Here's the drawing with two shaded views (mm, measured from the low corner). I have some questions. Coordinates: 2 decimals unless noted, no trailing zeros. Write each loop counter-clockwise with the first axis right and the second up, starting at its lowest first coordinate (ties: lowest second). Pieces come first, ordered by that corner, then holes.
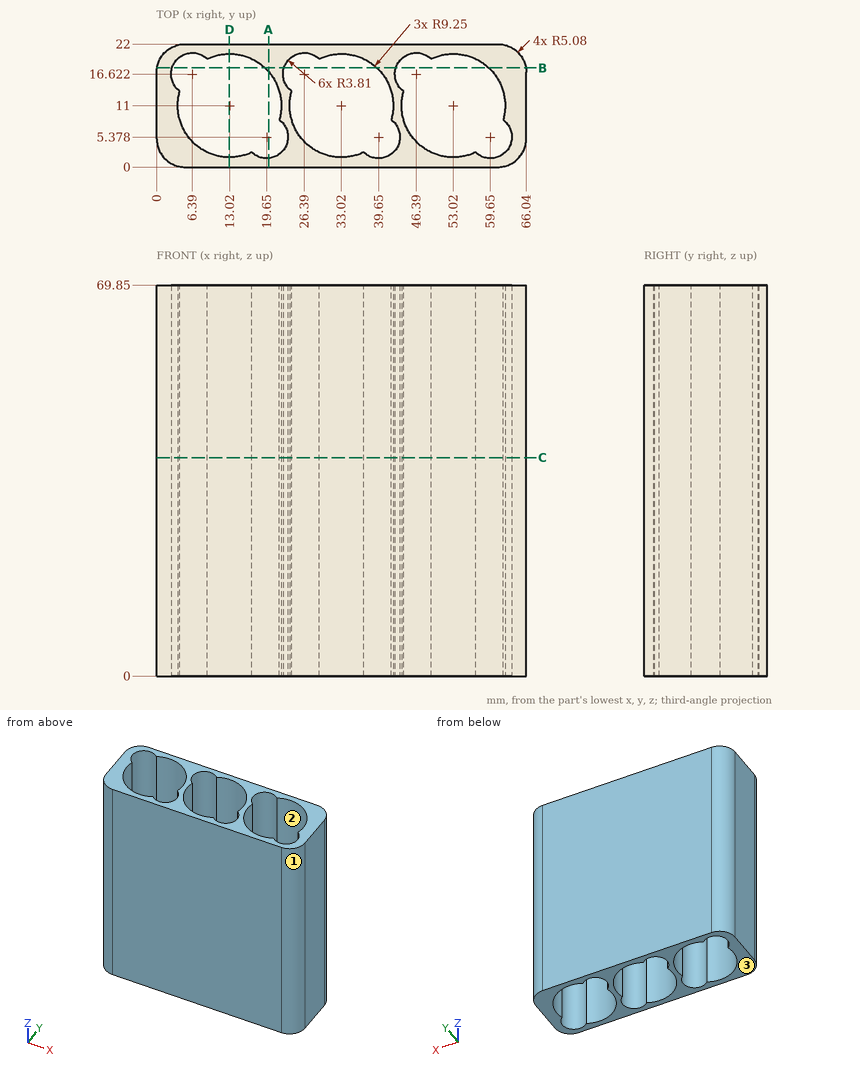
Item 1: I want a section at D-D, the plane x = 13. List the corners of the cut face in (y, z) for me.
Item 2: I want a section at A-A, the plane x = 20. List the corners of the cut face in (y, z) for me, then the cut area to 3 significant figures.
Item 3: If we mould it in two halves opening along X, with no side actions, what happens to the marked faces 1, 2 and 3? For each: released by +X, released by -X, zero draft, split by the parting line, or undercut.
Item 4: I want a section at C-C, the plane z = 39. List the corners of the cut face in (x, y) for me, then the cut area to 3 significant figures.
Item 5: I want a section at B-B, the plane y = 17.75. List the corners of the cut face in (x, z) for me, then the cut area to 3 significant figures.
Item 6: If I drill on line 1 along X through (y, z) = (10.75, 20.5); line 2 along X through (y, z) = (13.5, 38.5); line 3 along Y through (x, z) = (33, 34.5), over which ranges is the centre line in solid material (lowest first)?
Taken from the geometry:
1. outline: (0, 0) - (1.75, 0) - (1.75, 69.85) - (0, 69.85) - close; (20.25, 0) - (22, 0) - (22, 69.85) - (20.25, 69.85) - close
2. outline: (0, 0) - (1.58, 0) - (1.58, 69.85) - (0, 69.85) - close; (17.07, 0) - (22, 0) - (22, 69.85) - (17.07, 69.85) - close
2. area: 455 mm2
3. face 1: released by +X
3. face 2: undercut
3. face 3: zero draft
4. outline: (0, 5.08) arc R5.08 ccw to (5.08, 0) - (60.96, 0) arc R5.08 ccw to (66.04, 5.08) - (66.04, 16.92) arc R5.08 ccw to (60.96, 22) - (5.08, 22) arc R5.08 ccw to (0, 16.92) - close; hole (4.13, 13.55) arc R9.25 ccw to (16.99, 2.65) arc R3.81 ccw (long way) to (21.91, 8.45) arc R9.25 ccw to (9.05, 19.35) arc R3.81 ccw (long way) to start; hole (24.13, 13.55) arc R9.25 ccw to (36.99, 2.65) arc R3.81 ccw (long way) to (41.91, 8.45) arc R9.25 ccw to (29.05, 19.35) arc R3.81 ccw (long way) to start; hole (44.13, 13.55) arc R9.25 ccw to (56.99, 2.65) arc R3.81 ccw (long way) to (61.91, 8.45) arc R9.25 ccw to (49.05, 19.35) arc R3.81 ccw (long way) to start
4. area: 501 mm2
5. outline: (0.07, 0) - (2.75, 0) - (2.75, 69.85) - (0.07, 69.85) - close; (19.34, 0) - (22.75, 0) - (22.75, 69.85) - (19.34, 69.85) - close; (39.34, 0) - (42.75, 0) - (42.75, 69.85) - (39.34, 69.85) - close; (59.34, 0) - (65.97, 0) - (65.97, 69.85) - (59.34, 69.85) - close
5. area: 1,130 mm2
6. line 1: x = 0 to 3.77, 22.27 to 23.77, 42.27 to 43.77, 62.27 to 66.04
6. line 2: x = 0 to 4.11, 21.93 to 24.11, 41.93 to 44.11, 61.93 to 66.04
6. line 3: y = 0 to 1.75, 20.25 to 22
